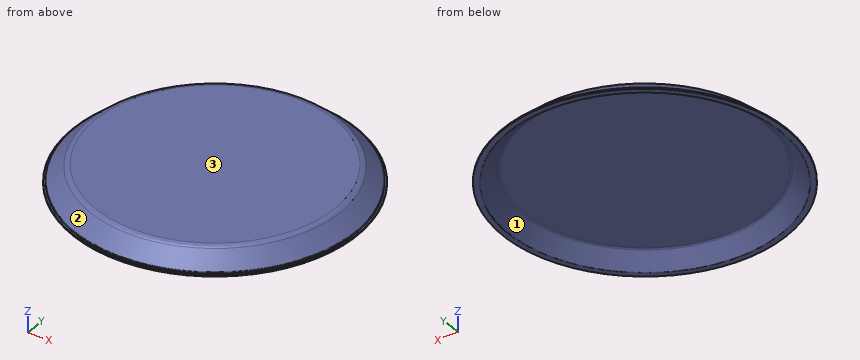
from build123d import *


with BuildPart() as part:
    # Sketch1 → Revolve1 (revolve)
    with BuildSketch(Plane(origin=(0, 0, 0), x_dir=(0, 0, -1), z_dir=(1, 0, 0))):
        with BuildLine():
            Line((0.199998156, 18.250858843), (0.368480901, 18.253649875))
            Line((0.368480901, 18.253649875), (0.368480901, 17.564198472))
            ThreePointArc((0.368480901, 17.564198472), (0.36191796, 17.528568202), (0.34309058, 17.497614721))
            Line((0.34309058, 17.497614721), (-1.298438714, 15.6582174))
            ThreePointArc((-1.298438714, 15.6582174), (-1.373748235, 15.534403473), (-1.4, 15.391882396))
            Line((-1.4, 15.391882396), (-1.4, 0))
            Line((-1.4, 0), (-2, 0))
            Line((-2, 0), (-2, 15.377593236))
            ThreePointArc((-2, 15.377593236), (-1.934370586, 15.733895926), (-1.746096785, 16.043430744))
            Line((-1.746096785, 16.043430744), (-0.029650113, 17.966775897))
            ThreePointArc((-0.029650113, 17.966775897), (0.003888132, 17.991368554), (0.044530144, 18.000191224))
            Line((0.044530144, 18.000191224), (0.199998156, 18.000858843))
            Line((0.199998156, 18.000858843), (0.199998156, 18.250858843))
        make_face()
    revolve(axis=Axis((0, 0, 10.644061054), (0, 0, -1)))


solid = part.part
Design review of the part built by this model. Coordinates are the model's own, in mm. Face numbers are marked on the shaded views. Round coordinates to 2 decimals unless told otherwise and drop trailing zeros. Write each loop counter-clockwise with the first axis right and the second up, starting at its lowest first coordinate (ties: lowest second). Pieces come first, ordered by that corner, then holes. Notation, with made-up numbers: (59.5, 47) -> (68.5, 47) arc R9 cw to (68.5, 54) -> close; hole circle Ø2 at (74, 11). An arc over 180 degrees is marked (long way). One line per item, written item: value. Start each with the question number.
Q1. Add section A-A (z = 0.85). Give the boundary of the cut face in (x, y).
Q2. Insertion check: P1, Ø5, axis at x = -6, y = -0.5, coming from the -Z side; P2, Ø6, axis at x = -13, y = -4, coming from the -Z side; P3, Ø1, axis at x = -1, z = 1, coming from the +Y side. Each pin has a flat end and moves straight along its axis. Give the tip position at first contact, or say it passes through.
Q3. The part is to be moulded in two halves that separate along Y. For the marked faces 1, 2 and 3, say which applies: pulls with the +Y half, pulls with the -Y half, needs draft (parallel to the pull), parting line crosses it, or undercut.
Q4. To check wall thickness, follow probe 1 along Z at (x, y) = (5.5, -11); probe 2 along X at (y, z) = (-1.5, 0.9); probe 3 along Y at (x, z) = (1.5, 0.15). State the ranges of each line that lie inside material, in increasing order.
Response:
1. outline: circle Ø34.1 at (0, 0); hole circle Ø32.32 at (0, 0)
2. P1: stops at z = 1.4
2. P2: stops at z = 0.46
2. P3: stops at y = 17.41
3. face 1: undercut
3. face 2: parting line crosses it
3. face 3: needs draft
4. probe 1: z = 1.4 to 2
4. probe 2: x = -16.93 to -16.03, 16.03 to 16.93
4. probe 3: y = -17.77 to -16.88, 16.88 to 17.77
